For this review, take the finished solid that the model builds, in its own axes (mm). Face numbers are marked on the shaded views. A direction names the side the tool comes from. Give positions to 0.01 mm unless a question says otherwise; leave off trailing zeros. Loops run counter-clockwise (first coordinate to the right, second up) from the corner with the lowest first, then second, coordinate; pieces in that order, holes last.
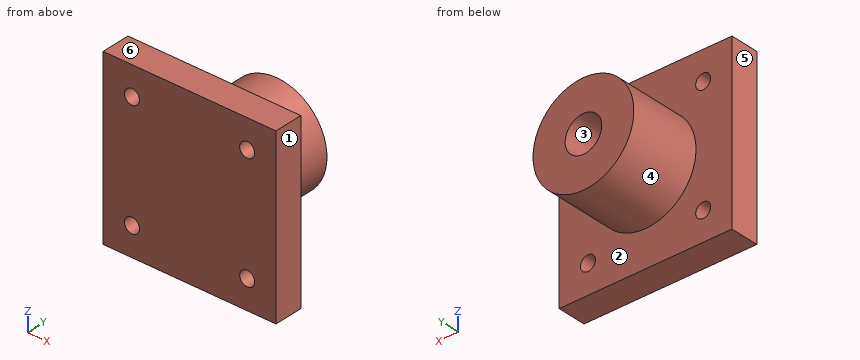
```python
from build123d import *

# Parameters (mm, degrees)
SKETCH1_W           = 60
SKETCH1_H           = 60
SKETCH1_R           = 2.6
BOSS_EXTRUDE1_DEPTH = 10
SKETCH2_R           = 17.5
SKETCH2_R_2         = 6.35889
BOSS_EXTRUDE2_DEPTH = 25


with BuildPart() as part:
    # Sketch1 → Boss-Extrude1 (new body)
    with BuildSketch(Plane(origin=(0, 0, 0), x_dir=(1, 0, 0), z_dir=(0, 1, 0))):
        Rectangle(SKETCH1_W, SKETCH1_H)
        with Locations(Location((-20, 20, 0), (0, 0, 270))):
            Circle(SKETCH1_R, mode=Mode.SUBTRACT)
        with Locations(Location((20, 20, 0), (0, 0, 270))):
            Circle(SKETCH1_R, mode=Mode.SUBTRACT)
        with Locations(Location((-20, -20, 0), (0, 0, 270))):
            Circle(SKETCH1_R, mode=Mode.SUBTRACT)
        with Locations(Location((20, -20, 0), (0, 0, 270))):
            Circle(SKETCH1_R, mode=Mode.SUBTRACT)
    extrude(amount=BOSS_EXTRUDE1_DEPTH)

    # Sketch2 → Boss-Extrude2 (add)
    with BuildSketch(Plane(origin=(0, 10, 0), x_dir=(1, 0, 0), z_dir=(0, 1, 0))):
        with Locations(Location((0, 0, 0), (0, 0, 270))):
            Circle(SKETCH2_R)
        with Locations(Location((0, 0, 0), (0, 0, 270))):
            Circle(SKETCH2_R_2, mode=Mode.SUBTRACT)
    extrude(amount=BOSS_EXTRUDE2_DEPTH)


solid = part.part
```
Q1. Consider section C-C on y = 6.5. Give the boundary of the cut face in (x, z).
Answers:
outline: (-30, -30) - (30, -30) - (30, 30) - (-30, 30) - close; hole circle Ø5.2 at (-20, -20); hole circle Ø5.2 at (-20, 20); hole circle Ø5.2 at (20, -20); hole circle Ø5.2 at (20, 20)
Q2. Machinability: for the marked faces 1 and 2, which of the approach directions +Z, -Z, +X, -X, +Y, -Y give a long, thin tool a straight path to every point of the face, cutting with its end or side? Answer none if there is none.
Answers:
face 1: +Z, -Z, +X, +Y, -Y
face 2: +Y
Q3. For pin 1 Ø1.5 at (x, y) = (-4, 20.5) entering from +Z; pin 2 Ø4 at (x, z) = (20, -20) entering from -Y; pin 3 Ø2 at (y, z) = (22, -15.5) entering from +X; pin 4 Ø6 at (x, y) = (-13.5, 31) entering from -Z, all flat-tipped, find the tip position at first contact; note any pin that passes through.
Answers:
pin 1: stops at z = 17.2
pin 2: passes through
pin 3: stops at x = 9.8
pin 4: stops at z = -14
Q4. Consider section A-A on z = 20. Give the boundary of the cut face in (x, y), plus the area to 3 significant figures.
Answers:
outline: (-30, 0) - (-22.6, 0) - (-22.6, 10) - (-30, 10) - close; (-17.4, 0) - (17.4, 0) - (17.4, 10) - (-17.4, 10) - close; (22.6, 0) - (30, 0) - (30, 10) - (22.6, 10) - close
area: 496 mm2
Q5. For probe 1 along X at (y, z) = (4.5, 20); probe 2 along Y at (x, z) = (-18, -22); probe 3 along X at (y, z) = (12, -1.5), list the stretches that pass through material, from the lowest coordinate up.
Answers:
probe 1: x = -30 to -22.6, -17.4 to 17.4, 22.6 to 30
probe 2: y = 0 to 10
probe 3: x = -17.44 to -6.18, 6.18 to 17.44
Q6. Mouldability with a two-part tool opening along Z and no side actions: class the marked faces 3, 4, 5 and 6 as +Z half, -Z half, draft (parallel to the pull), parting line (faces both ways), or undercut.
Answers:
face 3: undercut
face 4: parting line
face 5: draft
face 6: +Z half
Q7. Consider section B-B on x = -20. Give the boundary of the cut face in (y, z).
Answers:
outline: (0, -30) - (10, -30) - (10, -22.6) - (0, -22.6) - close; (0, -17.4) - (10, -17.4) - (10, 17.4) - (0, 17.4) - close; (0, 22.6) - (10, 22.6) - (10, 30) - (0, 30) - close
Q8. Consider section D-D on z = 0. Give the boundary of the cut face in (x, y).
Answers:
outline: (-30, 0) - (30, 0) - (30, 10) - (17.5, 10) - (17.5, 35) - (6.36, 35) - (6.36, 10) - (-6.36, 10) - (-6.36, 35) - (-17.5, 35) - (-17.5, 10) - (-30, 10) - close
